from build123d import *

# Parameters (mm, degrees)
SKETCH1_R           = 3
SKETCH1_R_2         = 1.5
BOSS_EXTRUDE1_DEPTH = 7.5
CUT_EXTRUDE1_REACH  = 70.715
SKETCH2_W           = 20.337315641
SKETCH2_H           = 5.5


with BuildPart() as part:
    # Sketch1 → Boss-Extrude1 (new, symmetric)
    with BuildSketch(Plane.XY):
        with BuildLine():
            Line((0, -5), (63.65524487, -5))
            ThreePointArc((63.65524487, -5), (65.064783801, -4.013030215), (64.619426284, -2.350933335))
            Line((64.619426284, -2.350933335), (51.928362829, 8.298133329))
            ThreePointArc((51.928362829, 8.298133329), (48.732145215, 8.718923361), (47, 6))
            Line((47, 6), (47, 2.491190702))
            ThreePointArc((47, 2.491190702), (46.188975519, 0.64799736), (44.282110643, 0.000703957))
            Line((44.282110643, 0.000703957), (10, 3))
            ThreePointArc((10, 3), (2.85176017, 7.632257918), (2.678290028, 16.148422208))
            ThreePointArc((2.678290028, 16.148422208), (0.935327464, 20.350467073), (-2.958378986, 17.997989735))
            ThreePointArc((-2.958378986, 17.997989735), (-4.206114513, 9.18048564), (-4.990396875, 0.30974026))
            ThreePointArc((-4.990396875, 0.30974026), (-3.643398228, -3.424273551), (0, -5))
        make_face()
        Circle(SKETCH1_R, mode=Mode.SUBTRACT)
        with Locations((50, 6)):
            Circle(SKETCH1_R_2, mode=Mode.SUBTRACT)
    extrude(amount=BOSS_EXTRUDE1_DEPTH, both=True)

    # Sketch2 → Cut-Extrude1 (cut, up to next)
    with BuildSketch(Plane(origin=(0, 0, 0), x_dir=(1, 0, 0), z_dir=(0, 1, 0)), mode=Mode.PRIVATE) as cut_extrude1_sk1:
        with Locations((54.450768463, 0)):
            Rectangle(SKETCH2_W, SKETCH2_H)
    cut_extrude1_tool1 = extrude(cut_extrude1_sk1.sketch, amount=CUT_EXTRUDE1_REACH, mode=Mode.PRIVATE) & part.part
    add(cut_extrude1_tool1.solids().sort_by_distance((54.450768, 0, 0))[0], mode=Mode.SUBTRACT)


solid = part.part
Source: CAD feature listing. Evaluate the final solid. Frame: model axes, mm. A direction names the side the tool comes from. Coordinates: 2 decimals unless noted, no trailing zeros. Order: outer loops, then holes, each group sorted by start corner. A loop starts at its lowest first (then second) coordinate and runs counter-clockwise, first axis right, second up. Notation, with made-up numbers: M 9.25,27.5 L 54.25,27.5 A22 cw 54.25,34.5 Z; hole C -16.5,77.25 d1. An arc over 180 degrees is marked long. Write each question's results on one line, items separated by ' | '. Start each with the question number.
1. Section A-A, the plane x = 50. Return the cut outline in (y, z).
2. Section C-C, the plane z = 0.25. Return the cut outline in (x, y), then the cut area to 3 significant figures.
3. Material intervals for L1, parallel to X at y = 6, z = -4.7; L2, parallel to Y at x = 0, z = 0.75; L3, parallel to Y at x = 50, z = 6.5, sorted ascending.
4. Reachability of faces 4 (the face through (31, -5, 0)), 5 (the face through (2.913, 7.524, 0.105)), 6 (the face through (47, 4, -5)), 7 (the face through (53, 0, 0)) from +Z, -Z, +X, -X, +Y, -Y: full face, straight path, thin tool, end or side. Return the list, or none.
5. Section D-D, the plane z = 4.25. Return the cut outline in (x, y), then the cut area to 3 significant figures.
6. Pin query (flat end, axial travel): pin 1 (1.1 mm diameter, centred on y = 5, z = -4, fed in from -X); pin 2 (4 mm diameter, centred on y = 7.5, z = -1, fed in from -X); pin 3 (1.1 mm diameter, centred on y = 4, z = 6, fed in from -X). Return the tip coordinate at first contact, or that it passes through.
7. Draft query along Z for faces 1 (the face through (58.36, 2.9, 3.44)), 2 (the face through (25, 1, -7.5)), 3 (the face through (53, 3, 2.75)). Return one class per face: +Z half, -Z half, draft (parallel to the pull), parting line (faces both ways), or undercut.
8. Section B-B, the plane y = 1. Return the cut outline in (x, z), then the cut area to 3 significant figures.
Solution:
1) outline: M -5,-7.5 L 4.5,-7.5 L 4.5,-2.75 L 0,-2.75 L 0,2.75 L 4.5,2.75 L 4.5,7.5 L -5,7.5 Z; M 7.5,-7.5 L 9,-7.5 L 9,-2.75 L 7.5,-2.75 Z; M 7.5,2.75 L 9,2.75 L 9,7.5 L 7.5,7.5 Z
2) outline: M -4.99,0.31 A5 ccw 0,-5 L 63.66,-5 A1.5 ccw 64.62,-2.35 L 61.82,0 L 44.71,0 A2.5 cw 44.28,0 L 10,3 A9.09 cw 2.68,16.15 A3 ccw long -2.96,18 A170 ccw Z; hole C 0,0 d6 | area: 526 mm²
3) L1: -4.54 to 4.01, 47 to 48.5, 51.5 to 54.67 | L2: -5 to -3, 3 to 20.5 | L3: -5 to 4.5, 7.5 to 9
4) face 4: +Z, -Z, +X, -X, -Y | face 5: +Z, -Z | face 6: +Z, -Z, +Y | face 7: +X, +Y
5) outline: M -4.99,0.31 A5 ccw 0,-5 L 63.66,-5 A1.5 ccw 64.62,-2.35 L 51.93,8.3 A3 ccw 47,6 L 47,2.49 A2.5 cw 44.28,0 L 10,3 A9.09 cw 2.68,16.15 A3 ccw long -2.96,18 A170 ccw Z; hole C 0,0 d6; hole C 50,6 d3 | area: 603 mm²
6) pin 1: x = -4.68 | pin 2: x = -4.59 | pin 3: x = -4.77
7) face 1: draft | face 2: -Z half | face 3: undercut
8) outline: M -4.95,-7.5 L -2.83,-7.5 L -2.83,7.5 L -4.95,7.5 Z; M 2.83,-7.5 L 32.86,-7.5 L 32.86,7.5 L 2.83,7.5 Z; M 46.51,-7.5 L 60.63,-7.5 L 60.63,-2.75 L 46.51,-2.75 Z; M 46.51,2.75 L 60.63,2.75 L 60.63,7.5 L 46.51,7.5 Z | area: 616 mm²
